Work out the finished part from the listing and answer in its coordinate system (mm). Face numbers are marked on the shaded views. Round coordinates to 2 decimals unless told otherwise and drop trailing zeros. Loops run counter-clockwise (first coordinate to the right, second up) from the corner with the lowest first, then second, coordinate; pieces in that order, holes last. Notation, with made-up numbers: (-3.75, -27) - (43.25, -27) arc R19 cw to (43.25, 4) - close; hole circle Ø9 at (39.5, 66). An arc over 180 degrees is marked (long way). Answer as CSV lines item,"result". Start each with the question number.
Q1. Section A-A on z = 0 is taken. Write down the section's boundary in (x, y).
Q2. Each of these flat-tipped pins is pushed along its axis until it touches: pin 1 Ø2.5 at (y, z) = (-2.5, -14) entering from -X; pin 2 Ø12.5 at (x, z) = (0, 0) entering from +Y; pin 3 Ø5 at (x, z) = (0, 11.358) entering from -Y. Where does it stop, or does it pass through?
Q3. Section D-D on y = -58.5 is taken. Write down the section's boundary in (x, z).
Q4. Section C-C on x = 0 is taken. Write down the section's boundary in (y, z).
Q5. Straight lines are drawn through the part: L1, parallel to X at y = -1.3, z = 0; L2, parallel to Y at x = 27, z = 0; L3, parallel to Y at x = -9, z = -15.5. For each, find the intervals that lie inside material, in ascending order. Write a range as [from, to].
Q6. Section B-B on x = -25 is taken. Write down the section's boundary in (y, z).
Q7. The mould has two halves that part along Y. Classify the marked faces 1, 2 and 3: +Y half, -Y half, draft (parallel to the pull), parting line (faces both ways), or undercut.
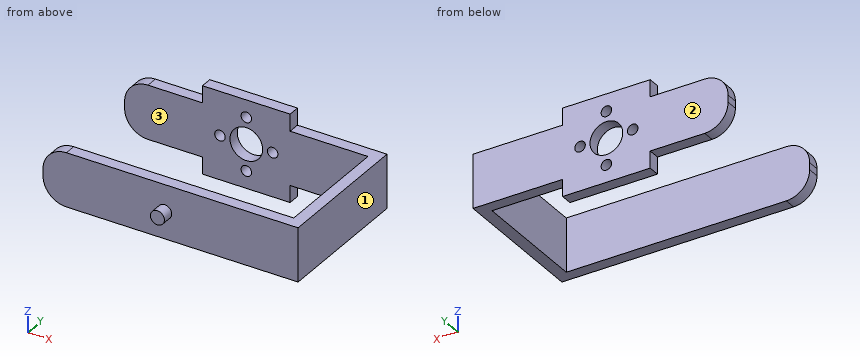
```python
from build123d import *

# Parameters (mm, degrees)
SKETCH1_W           = 33.32
SKETCH1_H           = 23
SKETCH1_R           = 2.25
SKETCH1_R_2         = 7
SKETCH1_H_2         = 11.5
BOSS_EXTRUDE2_DEPTH = 5
SKETCH1_3_W         = 5
SKETCH1_3_H         = 11.5
BOSS_EXTRUDE3_DEPTH = 60.8
SKETCH3_W           = 109.14
SKETCH3_H           = 23
BOSS_EXTRUDE4_DEPTH = 5
SKETCH4_R           = 3
BOSS_EXTRUDE5_DEPTH = 5
FILLET3_R           = 10


with BuildPart() as part:
    # Sketch1 → Boss-Extrude2 (new body)
    # profile 1 of 4: a face of its own
    with BuildSketch(Plane(origin=(0, 0, 0), x_dir=(1, 0, 0), z_dir=(0, 1, 0))):
        with Locations((-35.41, 0)):
            Rectangle(SKETCH1_W, SKETCH1_H)
    # profile 2 of 4: a face of its own
    with BuildSketch(Plane(origin=(0, 0, 0), x_dir=(1, 0, 0), z_dir=(0, 1, 0))):
        Polygon((18.75, 0), (18.75, 11.5), (18.75, 18.75), (-18.75, 18.75), (-18.75, 11.5), (-18.75, -11.5), (-18.75, -18.75), (18.75, -18.75), (18.75, -11.5), align=None)
        with Locations(Location((-11.26924292, 0, 0), (0, 0, 270))):
            Circle(SKETCH1_R, mode=Mode.SUBTRACT)
        with Locations(Location((0, -11.358, 0), (0, 0, 270))):
            Circle(SKETCH1_R, mode=Mode.SUBTRACT)
        with Locations(Location((0, 0, 0), (0, 0, 270))):
            Circle(SKETCH1_R_2, mode=Mode.SUBTRACT)
        with Locations(Location((11.26924292, 0, 0), (0, 0, 270))):
            Circle(SKETCH1_R, mode=Mode.SUBTRACT)
        with Locations(Location((0, 11.358, 0), (0, 0, 270))):
            Circle(SKETCH1_R, mode=Mode.SUBTRACT)
    # profile 3 of 4: a face of its own
    with BuildSketch(Plane(origin=(0, 0, 0), x_dir=(1, 0, 0), z_dir=(0, 1, 0))):
        with Locations((35.41, -5.75)):
            Rectangle(SKETCH1_W, SKETCH1_H_2)
    # profile 4 of 4: a face of its own
    with BuildSketch(Plane(origin=(0, 0, 0), x_dir=(1, 0, 0), z_dir=(0, 1, 0))):
        with Locations((35.41, 5.75)):
            Rectangle(SKETCH1_W, SKETCH1_H_2)
    extrude(amount=-BOSS_EXTRUDE2_DEPTH)

    # Sketch1_3 → Boss-Extrude3 (add)
    with BuildSketch(Plane(origin=(0, 0, 0), x_dir=(1, 0, 0), z_dir=(0, 1, 0))):
        with Locations((54.57, -5.75)):
            Rectangle(SKETCH1_3_W, SKETCH1_3_H)
        with Locations((54.57, 5.75)):
            Rectangle(SKETCH1_3_W, SKETCH1_3_H)
    extrude(amount=-BOSS_EXTRUDE3_DEPTH)

    # Sketch3 → Boss-Extrude4 (add)
    with BuildSketch(Plane.XZ.offset(60.8)):
        with Locations((2.5, 0)):
            Rectangle(SKETCH3_W, SKETCH3_H)
    extrude(amount=-BOSS_EXTRUDE4_DEPTH)

    # Sketch4 → Boss-Extrude5 (add)
    with BuildSketch(Plane.XZ.offset(60.8)):
        with Locations(Location((0, 0, 0), (0, 0, 90))):
            Circle(SKETCH4_R)
    extrude(amount=BOSS_EXTRUDE5_DEPTH)

    # Fillet3
    fillet3_edges = [part.edges().sort_by_distance(p)[0] for p in [
        (-52.07, -2.5, 11.5),
        (-52.07, -2.5, -11.5),
        (-52.07, -58.3, -11.5),
        (-52.07, -58.3, 11.5),
    ]]
    fillet(fillet3_edges, radius=FILLET3_R)


solid = part.part
```
Findings:
1,outline,"(-52.07, -60.8) - (-3, -60.8) - (-3, -65.8) - (3, -65.8) - (3, -60.8) - (57.07, -60.8) - (57.07, 0) - (13.52, 0) - (13.52, -5) - (52.07, -5) - (52.07, -55.8) - (-52.07, -55.8) - close; (-52.07, -5) - (-13.52, -5) - (-13.52, 0) - (-52.07, 0) - close; (-9.02, -5) - (-7, -5) - (-7, 0) - (-9.02, 0) - close; (7, -5) - (9.02, -5) - (9.02, 0) - (7, 0) - close"
2,pin 1,"stops at x = -18.75"
2,pin 2,"stops at y = -55.8"
2,pin 3,"stops at y = -60.8"
3,outline,"(-52.07, -1.5) arc R10 ccw to (-42.07, -11.5) - (57.07, -11.5) - (57.07, 11.5) - (-42.07, 11.5) arc R10 ccw to (-52.07, 1.5) - close"
4,outline,"(-65.8, -3) - (-60.8, -3) - (-60.8, -11.5) - (-55.8, -11.5) - (-55.8, 11.5) - (-60.8, 11.5) - (-60.8, 3) - (-65.8, 3) - close; (-5, -18.75) - (0, -18.75) - (0, -13.61) - (-5, -13.61) - close; (-5, -9.11) - (0, -9.11) - (0, -7) - (-5, -7) - close; (-5, 7) - (0, 7) - (0, 9.11) - (-5, 9.11) - close; (-5, 13.61) - (0, 13.61) - (0, 18.75) - (-5, 18.75) - close"
5,L1,"x = [-52.07, -13.52], [-9.02, -7], [7, 9.02], [13.52, 57.07]"
5,L2,"y = [-60.8, -55.8], [-5, 0]"
5,L3,"y = [-5, 0]"
6,outline,"(-60.8, -11.5) - (-55.8, -11.5) - (-55.8, 11.5) - (-60.8, 11.5) - close; (-5, -11.5) - (0, -11.5) - (0, 11.5) - (-5, 11.5) - close"
7,face 1,"draft"
7,face 2,"+Y half"
7,face 3,"undercut"
